Geometry check sheet. Reference: drawing and pictorial views, mm from the part's lowest x, y, z. A direction names the side the tool comes from. Give positions to 0.01 mm unless a question says otherwise; leave off trailing zeros. Loops run counter-clockwise (first coordinate to the right, second up) from the corner with the lowest first, then second, coordinate; pieces in that order, holes last. Notation, with made-up numbers: M 85,20.5 L 120,20.5 A36 ccw 120,58.5 Z; hole C -31,-4 d8. An arc over 180 degrees is marked long. Use CSV: the item, a comma, the result in double quotes.
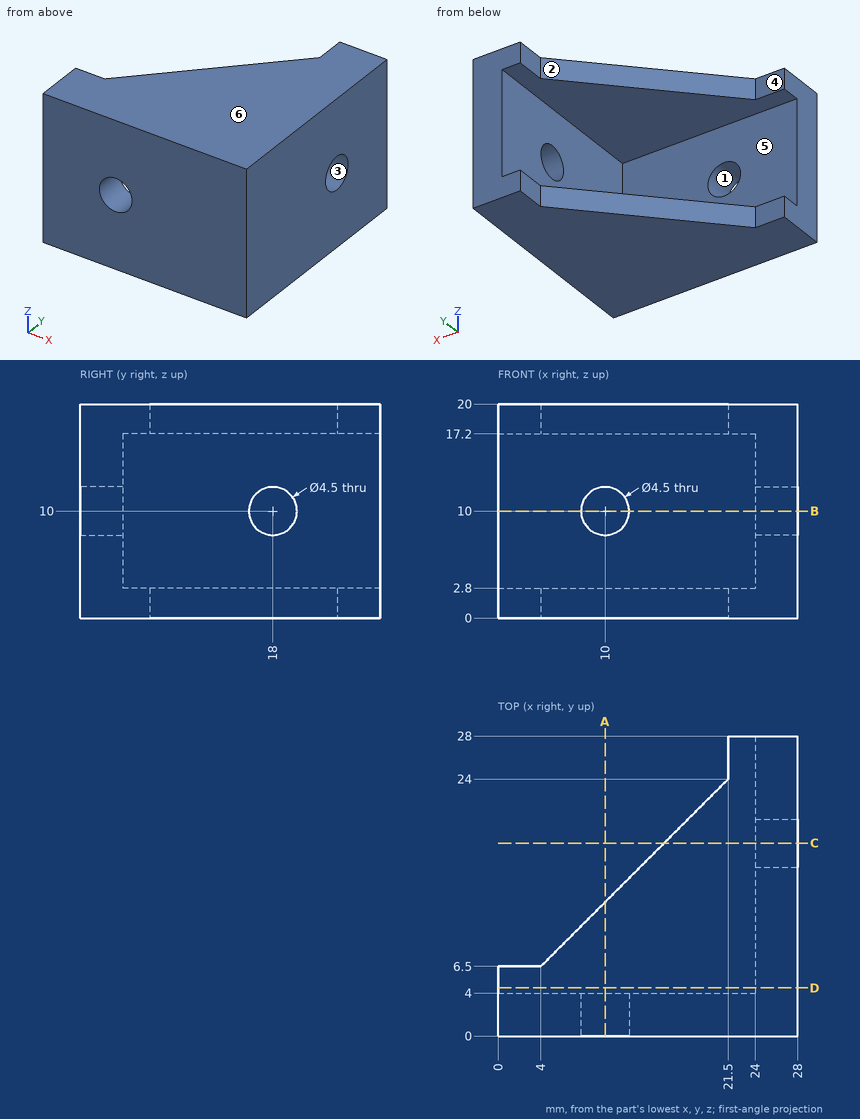
(1) Tool access check on the marked faces 4, 5 and 6. Record the directions out of +Z, -Z, +X, -X, +Y, -Y that give a thin tool (end or side, any length) a straight path to the whole face; none if there is none.
Calculated:
face 4,"+Z, -Z, -X, +Y"
face 5,"-X, +Y"
face 6,"+Z, +X, -X, +Y, -Y"
(2) Depth check by flat-ended pin: pin 1 Ø1.4 at (x, z) = (1, 2) entering from +Y; pin 2 Ø6 at (y, z) = (12.5, 12) entering from -X; pin 3 Ø0.8 at (y, z) = (25.5, 1) entering from -X. Enter the tip coordinate at first touch or a pass-through.
Calculated:
pin 1,"stops at y = 6.5"
pin 2,"stops at x = 24"
pin 3,"stops at x = 21.5"
(3) Mould release check, pull along X, two halves, no side actions. Record for the marked faces 1, 2 and 3: released by +X, released by -X, zero draft, split by the parting line, or undercut.
Calculated:
face 1,"undercut"
face 2,"released by -X"
face 3,"zero draft"
(4) Section check C-C on y = 18. Record the cut outline in (x, z), plus the area to 3 significant figures.
Calculated:
outline,"M 15.5,0 L 28,0 L 28,7.75 L 24,7.75 L 24,2.8 L 15.5,2.8 Z; M 15.5,17.2 L 24,17.2 L 24,12.25 L 28,12.25 L 28,20 L 15.5,20 Z"
area,"110 mm²"
(5) Section check D-D on y = 4.5. Record the cut outline in (x, z).
Calculated:
outline,"M 0,0 L 28,0 L 28,20 L 0,20 L 0,17.2 L 24,17.2 L 24,2.8 L 0,2.8 Z"
(6) Section check A-A on x = 10. Record the cut outline in (y, z).
Calculated:
outline,"M 0,0 L 12.5,0 L 12.5,2.8 L 4,2.8 L 4,7.75 L 0,7.75 Z; M 0,12.25 L 4,12.25 L 4,17.2 L 12.5,17.2 L 12.5,20 L 0,20 Z"
(7) Section check B-B on z = 10. Record the cut outline in (x, y), plus the area to 3 significant figures.
Calculated:
outline,"M 0,0 L 7.75,0 L 7.75,4 L 0,4 Z; M 12.25,0 L 28,0 L 28,15.75 L 24,15.75 L 24,4 L 12.25,4 Z; M 24,20.25 L 28,20.25 L 28,28 L 24,28 Z"
area,"172 mm²"
(8) Scan lines: L1, parallel to Z at x = 7.25, y = 4.75; L2, parallel to Y at x = 25.6, z = 10; L3, parallel to X at y = 2, z = 10. Record each from-to range of solid material in increasing order. Write a range as from..to.
Calculated:
L1,"z = 0..2.8, 17.2..20"
L2,"y = 0..15.75, 20.25..28"
L3,"x = 0..7.75, 12.25..28"
